```python
from build123d import *

# Parameters (mm, degrees)
F1_DEPTH     = 5
F0_R         = 1.75
F2_DEPTH     = 20
F3_R         = 3.25
F4_DEPTH     = 15
F5_R         = 1.35
F5_W         = 2.6
F5_H         = 6
F5_W_2       = 5
F6_DEPTH     = 5
F7_DEPTH     = 10
F8_R         = 3
F9_R         = 5
F10_T1_DEPTH = 14.8533585862
F11_R        = 1
F12_R        = 5
F13_R        = 5
F14_R        = 10


# Not quite as in the source:
# - a fillet or chamfer that OpenCascade refuses, or shapes differently, is made with other operations: its cross-section is extruded or revolved along the edge and cut away or added


with BuildPart() as f1:
    # F0 (on Right) → F1 (new body)
    with BuildSketch(Plane.YZ):
        Polygon((-15, -15), (-15, 0), (-15, 15), (-18, 15), (-18, 0), (-18, -18), (0, -18), (0, -15), align=None)
        with BuildLine():
            Line((3.7889535467, -15), (0, -15))
            Line((0, -15), (0, -18))
            ThreePointArc((0, -18), (1.9315685392, -16.546846326), (3.7889535467, -15))
        make_face()
    extrude(amount=F1_DEPTH)

    # F0 (on Right) → F2 (join)
    with BuildSketch(Plane.YZ):
        with BuildLine():
            Line((-15, 15), (-15, 0))
            Line((-15, 0), (-15, -15))
            Line((-15, -15), (0, -15))
            Line((0, -15), (3.7889535467, -15))
            ThreePointArc((3.7889535467, -15), (14.5947925758, -1.4591648304), (20, 15))
            Line((20, 15), (-15, 15))
        make_face()
        Circle(F0_R, mode=Mode.SUBTRACT)
        Polygon((-15, -15), (-15, 0), (-15, 15), (-18, 15), (-18, 0), (-18, -18), (0, -18), (0, -15), align=None)
        with BuildLine():
            Line((3.7889535467, -15), (0, -15))
            Line((0, -15), (0, -18))
            ThreePointArc((0, -18), (1.9315685392, -16.546846326), (3.7889535467, -15))
        make_face()
    extrude(amount=-F2_DEPTH)

    # F3 (on face) → F4 (join)
    with BuildSketch(Plane(origin=(-20, 0, 0), x_dir=(0, -1, 0), z_dir=(-1, 0, 0))):
        with BuildLine():
            Line((18, -18), (18, 15))
            Line((18, 15), (-20, 15))
            ThreePointArc((-20, 15), (-13.3934629181, -3.5566441928), (0, -18))
            Line((0, -18), (18, -18))
        make_face()
        Circle(F3_R, mode=Mode.SUBTRACT)
    extrude(amount=F4_DEPTH)

    # F5 (on face) → F6 (cut)
    with BuildSketch(Plane(origin=(-35, 0, 0), x_dir=(0, -1, 0), z_dir=(-1, 0, 0))):
        with Locations((-10.5, 12)):
            Circle(F5_R)
        with Locations((10.5, 12)):
            Circle(F5_R)
        with Locations((3.8, 12)):
            Rectangle(F5_W, F5_H)
        with BuildLine():
            Line((2.5, 2.0766559657), (2.5, 9))
            Line((2.5, 9), (-2.5, 9))
            Line((-2.5, 9), (-2.5, 2.0766559657))
            ThreePointArc((-2.5, 2.0766559657), (0, 3.25), (2.5, 2.0766559657))
        make_face()
        with Locations((0, 12)):
            Rectangle(F5_W_2, F5_H)
        with Locations((-3.8, 12)):
            Rectangle(F5_W, F5_H)
        with BuildLine():
            Line((18, 1), (3.0923292192, 1))
            ThreePointArc((3.0923292192, 1), (3.2103403217, 0.5061768651), (3.25, 0))
            ThreePointArc((3.25, 0), (3.0567548152, -1.1039701083), (2.5, -2.0766559657))
            Line((2.5, -2.0766559657), (2.5, -4))
            Line((2.5, -4), (18, -4))
            Line((18, -4), (18, 1))
        make_face()
        with BuildLine():
            ThreePointArc((2.5, -2.0766559657), (0, -3.25), (-2.5, -2.0766559657))
            Line((-2.5, -2.0766559657), (-2.5, -4))
            Line((-2.5, -4), (0, -4))
            Line((0, -4), (2.5, -4))
            Line((2.5, -4), (2.5, -2.0766559657))
        make_face()
    extrude(amount=-F6_DEPTH, mode=Mode.SUBTRACT)

    # F7 (cut): faces of the model
    f7_faces = [f1.faces().sort_by_distance(p)[0] for p in [
        (-30, 10.5, 12),
        (-30, -10.5, 12),
    ]]
    extrude(f7_faces, amount=-F7_DEPTH, mode=Mode.SUBTRACT)

    # F8
    f8_edges = [f1.edges().sort_by_distance(p)[0] for p in [
        (2.5, -15, -15),
    ]]
    fillet(f8_edges, radius=F8_R)

    # F9
    f9_edges = [f1.edges().sort_by_distance(p)[0] for p in [
        (-15, -18, -18),
    ]]
    fillet(f9_edges, radius=F9_R)

    # F10: fillet of radius 5 on 1 edges, made by hand

    # F10_s2 → F10_t1 (join)
    with BuildSketch(Plane.YZ.offset(-35)):
        with BuildLine():
            ThreePointArc((-1.4413434345, -4), (0.7514538853, -3.4935108673), (2.5, -2.0766559657))
            Line((2.5, -2.0766559657), (2.5, -4))
            Line((2.5, -4), (-1.4413434345, -4))
        make_face()
    extrude(amount=F10_T1_DEPTH)

    # F11
    f11_edges = [f1.edges().sort_by_distance(p)[0] for p in [
        (-32.5, 2.5, 9),
        (-32.5, -2.5, 9),
    ]]
    fillet(f11_edges, radius=F11_R)

    # F12
    f12_edges = [f1.edges().sort_by_distance(p)[0] for p in [
        (-17.5, 20, 15),
    ]]
    fillet(f12_edges, radius=F12_R)

    # F13
    f13_edges = [f1.edges().sort_by_distance(p)[0] for p in [
        (-15, -18, 15),
    ]]
    fillet(f13_edges, radius=F13_R)

    # F14
    f14_edges = [f1.edges().sort_by_distance(p)[0] for p in [
        (-15, 0, -18),
    ]]
    fillet(f14_edges, radius=F14_R)


solid = f1.part
```
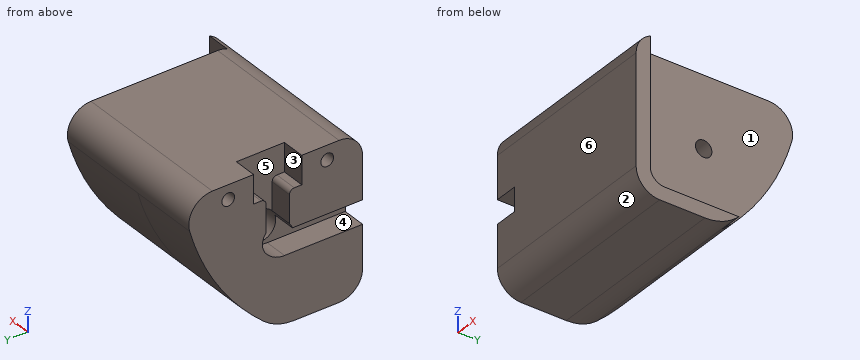
CAD build for the part. Positions are in the model's coordinates, mm. Face numbers are marked on the shaded views. A direction names the side the tool comes from. Give positions to 0.01 mm unless a question says otherwise; leave off trailing zeros. Order: outer loops, then holes, each group sorted by start corner. A loop starts at its lowest first (then second) coordinate and runs counter-clockwise, first axis right, second up. Notation, with made-up numbers: M -11,88.25 L 19,88.25 A12 ccw 19,97.25 Z; hole C 68.25,-2 d2. An arc over 180 degrees is marked long. Put each result on its own line as item: value. Start each with the question number.
(1) Mould opens along Y. For the marked faces 4, 5 and 6 say: +Y half, -Y half, draft (parallel to the pull), parting line (faces both ways), or undercut.
(2) Saw through at B-B, the plane x = -10. Write the cut outline in (y, z), then the cut area to 3 significant figures.
(3) Drill centre lines: line 1 along Y through (x, z) = (-26, 13); line 2 along Z through (x, y) = (-27.75, -10.5); line 3 along X through (y, z) = (-2, -5.5). Where is each one in solid material? Low to high.
(4) Saw through at A-A, the plane x = -32. Write the cut outline in (y, z), then the cut area to 3 significant figures.
(5) Saw through at D-D, the plane z = 0. Write the cut outline in (x, y), then the cut area to 3 significant figures.
(6) Flat gauge pins, fed straight in: pin 1 Ø4 at (x, z) = (-32.5, 4.5) entering from +Y; pin 2 Ø5 at (y, z) = (0.5, 1) entering from -X; pin 3 Ø2 at (y, z) = (-1.5, -5) entering from +X; pin 4 Ø5.5 at (x, z) = (-31.5, 13.5) entering from -Y. Where does each tip first touch, or does it go through?
(7) Which spindle directions (+Z, -Z, +X, -X, +Y, -Y) get a long thin tool onto all of the face, cutting with end or side? Do the marked faces 1, 2 and 3. Say none if no direction does.
(8) Saw through at C-C, the plane y = -10.5. Write the cut outline in (x, z).
Check result:
1. face 4: draft
1. face 5: undercut
1. face 6: -Y half
2. outline: M -18,-13 A5 ccw -13,-18 L -3.41,-18 A10 ccw 3.02,-15.66 A48.89 ccw 18.68,8.66 A5 ccw 13.86,15 L -13,15 A5 ccw -18,10 Z; hole C 0,0 d3.5
2. area: 996 mm2
3. line 1: y = -17 to -11.41, -9.59 to 9.59, 11.41 to 17.86
3. line 2: z = -18 to 10.65, 13.35 to 15
3. line 3: x = -35 to 0
4. outline: M -18,-13 A5 ccw -13,-18 L -3.41,-18 A10 ccw 3.02,-15.66 A48.89 ccw 18.68,8.66 A5 ccw 13.86,15 L 5.1,15 L 5.1,9 L 3.5,9 A1 ccw 2.5,8 L 2.5,2.08 A3.25 cw 2.5,-2.08 A5 cw -1.44,-4 L -18,-4 Z; M -18,1 L -3.09,1 A3.25 cw -2.5,2.08 L -2.5,8 A1 ccw -3.5,9 L -5.1,9 L -5.1,15 L -13,15 A5 ccw -18,10 Z; hole C -10.5,12 d2.7; hole C 10.5,12 d2.7
4. area: 790 mm2
5. outline: M -35,3.25 L -20,3.25 L -20,1.75 L 0,1.75 L 0,15.35 L -35,15.35 Z; M -30,-18 L 5,-18 L 5,-15 L 0,-15 L 0,-1.75 L -20,-1.75 L -20,-3.25 L -30,-3.25 Z
5. area: 941 mm2
6. pin 1: stops at y = 18.02
6. pin 2: stops at x = -35
6. pin 3: stops at x = 0
6. pin 4: stops at y = -17.94
7. face 1: +Z, +X, +Y
7. face 2: -Z, +X, -X, -Y
7. face 3: +Z, -X
8. outline: M -35,-18 L 5,-18 L 5,-15 L 0,-15 L 0,15 L -35,15 L -35,13.35 L -20,13.35 L -20,10.65 L -35,10.65 L -35,1 L -30,1 L -30,-4 L -35,-4 Z
